Verification items for the finished model (mm, model axes). A direction names the side the tool comes from. Round coordinates to 2 decimals unless told otherwise and drop trailing zeros. Order: outer loops, then holes, each group sorted by start corner. A loop starts at its lowest first (then second) coordinate and runs counter-clockwise, first axis right, second up. Notation, with made-up numbers: (-19.75, -14) -> (2.25, -14) arc R13 ccw to (2.25, 2) -> close; hole circle Ø4 at (16, -13). An arc over 180 degrees is marked (long way). Return JSON: item names as keys, results as strings. Group by question number.
Item 1: Sectioned sample at B-B on y = 0. Record the cut outline in (x, z), plus the area to 3 significant figures.
Item 2: Sectioned sample at D-D on z = 4.25. Give the number of separate pieces and of enclosed holes in the cut face, plus the area to 3 significant figures.
Item 3: Access from +Z, -Z, +X, -X, +Y, -Y to the whole of each face (thin tool, end or side, straight path). Record for faces 1 (the flat face through (3, -28, 2)), 2 (the flat face through (-10, 1, 5)), 3 (the flat face through (25.963, -15.03, 2.465)).
Item 4: Depth check by flat-ended pin: pin 1 Ø1.5 at (x, z) = (0.5, 1.5) entering from +Y; pin 2 Ø2.5 at (x, z) = (0, 3) entering from -Y; pin 3 Ø1 at (x, z) = (13, 1) entering from -Y. Enter the tip coordinate at first touch or a pass-through.
Item 5: Scan lines: probe 1 along Y at (x, z) = (0, 1.7); probe 2 along X at (y, z) = (-14.5, 0.9); probe 3 along X at (y, z) = (13, 1.55). Record each from-to range of solid material in increasing order. Write a range as from..to.
Item 6: Sectioned sample at A-A on x = 0. Record the cut outline in (y, z).
Item 7: Sectioned sample at C-C on y = 35. Record the cut outline in (x, z), plus the area to 3 significant figures.
Item 8: Draft check along X on faces 4 (the flat face through (-10, 1, 0)), 5 (the flat face through (34.624, -20.03, 2.465)). Enter one of: pulls with the +X half, pulls with the -X half, needs draft (parallel to the pull), parting line crosses it, or undercut.
```python
from build123d import *

# Parameters (mm, degrees)
ESQUISSE1_R        = 1.5
ESQUISSE1_W        = 5
ESQUISSE1_H        = 5
BOSS_EXTRU_1_DEPTH = 5
FILLET1_R          = 2


with BuildPart() as part:
    # Esquisse1 → Boss.-Extru.1 (new body)
    with BuildSketch(Plane.XY):
        with BuildLine():
            Line((-3, -6.9828361), (-3, -49.909918854))
            ThreePointArc((-3, -49.909918854), (0, 50), (3, -49.909918854))
            Line((3, -49.909918854), (3, -6.9828361))
            ThreePointArc((3, -6.9828361), (0, 7.6), (-3, -6.9828361))
        make_face()
        with Locations((14.142135624, 14.142135624)):
            Circle(ESQUISSE1_R, mode=Mode.SUBTRACT)
        with Locations(Location((14.142135624, -14.142135624, 0), (0, 0, 180))):
            Circle(ESQUISSE1_R, mode=Mode.SUBTRACT)
        with Locations(Location((-14.142135624, 14.142135624, 0), (0, 0, 180))):
            Circle(ESQUISSE1_R, mode=Mode.SUBTRACT)
        with Locations((-14.142135624, -14.142135624)):
            Circle(ESQUISSE1_R, mode=Mode.SUBTRACT)
        with Locations((0, 35)):
            Circle(ESQUISSE1_R, mode=Mode.SUBTRACT)
        with Locations((-30.310889132, -17.5)):
            Circle(ESQUISSE1_R, mode=Mode.SUBTRACT)
        with Locations((30.310889132, -17.5)):
            Circle(ESQUISSE1_R, mode=Mode.SUBTRACT)
        with Locations((0, 27.5)):
            Rectangle(ESQUISSE1_W, ESQUISSE1_H, mode=Mode.SUBTRACT)
        with Locations((0, 42.5)):
            Rectangle(ESQUISSE1_W, ESQUISSE1_H, mode=Mode.SUBTRACT)
        Polygon((-35.891016151, -17.834936491), (-40.22114317, -20.334936491), (-37.72114317, -24.665063509), (-33.391016151, -22.165063509), align=None, mode=Mode.SUBTRACT)
        Polygon((-27.230762114, -12.834936491), (-22.900635095, -10.334936491), (-20.400635095, -14.665063509), (-24.730762114, -17.165063509), align=None, mode=Mode.SUBTRACT)
        Polygon((27.230762114, -12.834936491), (22.900635095, -10.334936491), (20.400635095, -14.665063509), (24.730762114, -17.165063509), align=None, mode=Mode.SUBTRACT)
        Polygon((35.891016151, -17.834936491), (40.22114317, -20.334936491), (37.72114317, -24.665063509), (33.391016151, -22.165063509), align=None, mode=Mode.SUBTRACT)
    extrude(amount=BOSS_EXTRU_1_DEPTH)

    # Fillet1
    fillet1_edges = [part.edges().sort_by_distance(p)[0] for p in [
        (-3, -6.9828361, 2.5),
        (-3, -49.909918854, 2.5),
        (3, -49.909918854, 2.5),
        (3, -6.9828361, 2.5),
    ]]
    fillet(fillet1_edges, radius=FILLET1_R)


solid = part.part
```
Recorded:
{
 "1": {"outline": "(-50, 0) -> (-7.6, 0) -> (-7.6, 5) -> (-50, 5) -> close; (7.6, 0) -> (50, 0) -> (50, 5) -> (7.6, 5) -> close", "area": "424 mm²"},
 "2": {"separate pieces": "1", "enclosed holes": "13", "area": "7,220 mm²"},
 "3": {"face 1": "+Z, -Z, -Y", "face 2": "+Z, +X, -X, +Y, -Y", "face 3": "+Z, -Z"},
 "4": {"pin 1": "y = 50", "pin 2": "y = 7.5", "pin 3": "y = -48.41"},
 "5": {"probe 1": "7.6..25, 30..33.5, 36.5..40, 45..50", "probe 2": "-47.85..-26.27, -20.5..-15.6, -12.69..-3, 3..12.69, 15.6..20.5, 26.27..47.85", "probe 3": "-48.28..-15.11, -13.17..13.17, 15.11..48.28"},
 "6": {"outline": "(7.6, 0) -> (25, 0) -> (25, 5) -> (7.6, 5) -> close; (30, 0) -> (33.5, 0) -> (33.5, 5) -> (30, 5) -> close; (36.5, 0) -> (40, 0) -> (40, 5) -> (36.5, 5) -> close; (45, 0) -> (50, 0) -> (50, 5) -> (45, 5) -> close"},
 "7": {"outline": "(-35.71, 0) -> (-1.5, 0) -> (-1.5, 5) -> (-35.71, 5) -> close; (1.5, 0) -> (35.71, 0) -> (35.71, 5) -> (1.5, 5) -> close", "area": "342 mm²"},
 "8": {"face 4": "needs draft", "face 5": "undercut"}
}
